Verification items for this drawing (mm, ordinates from the low corner). A direction names the side the tool comes from. Round coordinates to 2 decimals unless told otherwise and drop trailing zeros. Order: outer loops, then holes, each group sorted by start corner. A loop starts at its lowest first (then second) coordinate and runs counter-clockwise, first axis right, second up. Notation, with made-up numbers: (10.25, -19.5) -> (38.25, -19.5) arc R23 ccw to (38.25, 10.5) -> close; hole circle Ø7 at (10, 85). An arc over 180 degrees is marked (long way). Answer in a Markdown table with one row per item.
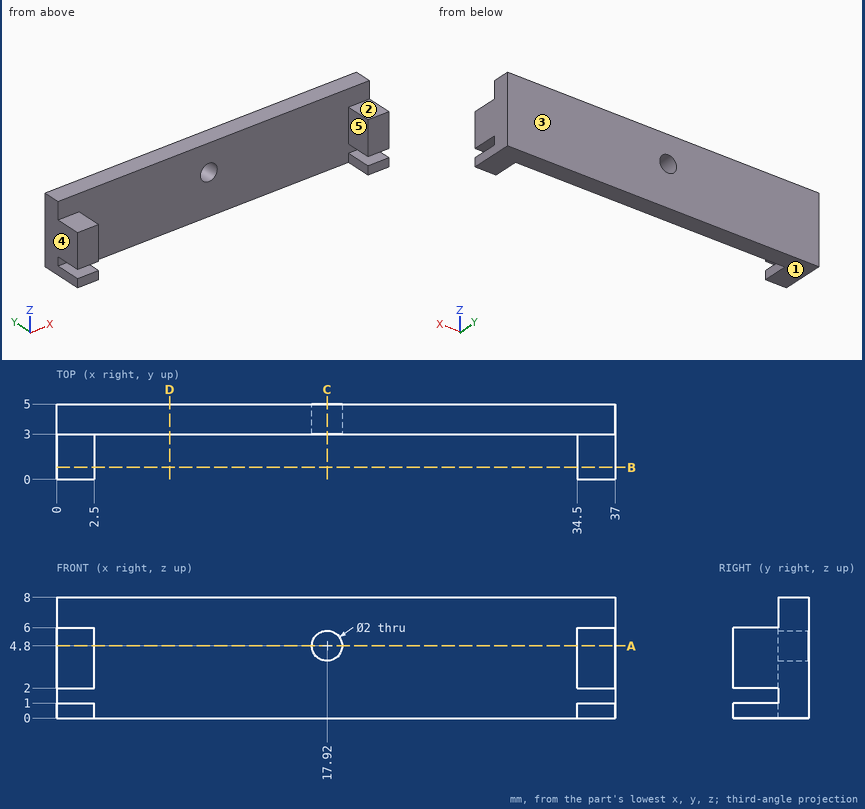
Item 1: Cross-section at A-A (z = 4.8). Record the boundary of the cut face in (x, y).
Result sheet:
| item | result |
|---|---|
| outline | (0, 0) -> (2.5, 0) -> (2.5, 3) -> (16.92, 3) -> (16.92, 5) -> (0, 5) -> close; (18.92, 3) -> (34.5, 3) -> (34.5, 0) -> (37, 0) -> (37, 5) -> (18.92, 5) -> close |
Item 2: Mould release check, pull along X, two halves, no side actions. Record for the marked faces 3, 4 and 5: pulls with the +X half, pulls with the -X half, needs draft (parallel to the pull), parting line crosses it, or undercut.
Result sheet:
| item | result |
|---|---|
| face 3 | needs draft |
| face 4 | pulls with the -X half |
| face 5 | undercut |
Item 3: Depth check by flat-ended pin: P1, Ø1.2, axis at x = 35.5, y = 1.5, coming from the +Z side. Enter the tip coordinate at first touch or a pass-through.
Result sheet:
| item | result |
|---|---|
| P1 | stops at z = 6 |
Item 4: Cross-section at B-B (y = 0.8). Record the boundary of the cut face in (x, z), and give its area (3 significant figures).
Result sheet:
| item | result |
|---|---|
| outline | (0, 0) -> (2.5, 0) -> (2.5, 1) -> (0, 1) -> close; (0, 2) -> (2.5, 2) -> (2.5, 6) -> (0, 6) -> close; (34.5, 0) -> (37, 0) -> (37, 1) -> (34.5, 1) -> close; (34.5, 2) -> (37, 2) -> (37, 6) -> (34.5, 6) -> close |
| area | 25.0 mm^2 |
Item 5: Scan lines: line 1 (X direction, y = 2.9, z = 4.25); line 2 (X direction, y = 3.75, z = 4.8); line 3 (Z direction, x = 17.92, y = 4.45). Record each from-to range of solid material in increasing order. Write a range as [from, to].
Result sheet:
| item | result |
|---|---|
| line 1 | x = [0, 2.5], [34.5, 37] |
| line 2 | x = [0, 16.92], [18.92, 37] |
| line 3 | z = [0, 3.8], [5.8, 8] |
Item 6: Cross-section at D-D (x = 7.5). Record the boundary of the cut face in (y, z), and give its area (3 significant figures).
Result sheet:
| item | result |
|---|---|
| outline | (3, 0) -> (5, 0) -> (5, 8) -> (3, 8) -> close |
| area | 16.0 mm^2 |
Item 7: Cross-section at C-C (x = 17.92). Record the boundary of the cut face in (y, z), and give its area (3 significant figures).
Result sheet:
| item | result |
|---|---|
| outline | (3, 0) -> (5, 0) -> (5, 3.8) -> (3, 3.8) -> close; (3, 5.8) -> (5, 5.8) -> (5, 8) -> (3, 8) -> close |
| area | 12.0 mm^2 |
Item 8: Set-up check for the marked faces 1 and 2: record each of +Z, -Z, +X, -X, +Y, -Y from which the full face is reachable in a straight line by a thin tool's end or side.
Result sheet:
| item | result |
|---|---|
| face 1 | -Z, +X, -X, +Y, -Y |
| face 2 | +Z, +X, -X, -Y |
